Can you work these out from the model? Positions are in its coordinate system, mm. Round coordinates to 2 decimals unless told otherwise and drop trailing zeros. Loops run counter-clockwise (first coordinate to the right, second up) from the corner with the lowest first, then second, coordinate; pieces in that order, holes last.
```python
from build123d import *

# Parameters (mm, degrees)
F1_DEPTH = 14
F2_R     = 8
F2_R_2   = 3.25
F3_DEPTH = 14.001


with BuildPart() as f1:
    # F0 (on Front) → F1 (new body)
    with BuildSketch(Plane.XZ):
        with BuildLine():
            Line((-46.5, -24.5), (46.5, -24.5))
            Line((46.5, -24.5), (46.5, 19.5))
            ThreePointArc((46.5, 19.5), (45.035534, 23.035534), (41.5, 24.5))
            Line((41.5, 24.5), (-41.5, 24.5))
            ThreePointArc((-41.5, 24.5), (-45.035534, 23.035534), (-46.5, 19.5))
            Line((-46.5, 19.5), (-46.5, -24.5))
        make_face()
    extrude(amount=F1_DEPTH)

    # F2 (on face) → F3 (cut, through all)
    with BuildSketch(Plane.XZ.offset(14)):
        Circle(F2_R)
        with Locations((-17, -6)):
            Circle(F2_R_2)
        with Locations((-25, 16)):
            Circle(F2_R_2)
        with Locations((25, 16)):
            Circle(F2_R_2)
        with Locations((17, -6)):
            Circle(F2_R_2)
    extrude(amount=-F3_DEPTH, mode=Mode.SUBTRACT)


solid = f1.part
```
(1) We'd pull the mould along Z, two halves only. Please class faces 1 (the cylindrical face through (24.577, -7.098, 19.222)), 2 (the cylindrical face through (-45, -6.9, 23.07)), 3 (the flat face through (46.5, -7, -3)), 4 (the cylindrical face through (-20.247, -7.098, -5.857)): released by +Z, released by -Z, zero draft, split by the parting line, or undercut.
(2) Suppose I cut it at A-A (x = -25). Write out the boundary of the cut face in (y, z).
(3) Suppose I cut it at C-C (z = -6). Write out the boundary of the cut face in (x, y), then the cut area to 3 significant figures.
(4) Suppose I cut it at D-D (z = 2.5). Write out the boundary of the cut face in (x, y).
(5) If I drill on line 1 (Z direction, x = -25, y = -11); line 2 (Z direction, x = -17, y = -4.75); line 3 (X direction, y = -3, z = 17.5), over which ranges is the centre line in solid material (lowest first)?
(6) Suppose I cut it at B-B (y = -5.5). Write out the boundary of the cut face in (x, z), then the cut area to 3 significant figures.
Check result:
1. face 1: undercut
1. face 2: released by +Z
1. face 3: zero draft
1. face 4: undercut
2. outline: (-14, -24.5) - (0, -24.5) - (0, 12.75) - (-14, 12.75) - close; (-14, 19.25) - (0, 19.25) - (0, 24.5) - (-14, 24.5) - close
3. outline: (-46.5, -14) - (-20.25, -14) - (-20.25, 0) - (-46.5, 0) - close; (-13.75, -14) - (-5.29, -14) - (-5.29, 0) - (-13.75, 0) - close; (5.29, -14) - (13.75, -14) - (13.75, 0) - (5.29, 0) - close; (20.25, -14) - (46.5, -14) - (46.5, 0) - (20.25, 0) - close
3. area: 972 mm2
4. outline: (-46.5, -14) - (-7.6, -14) - (-7.6, 0) - (-46.5, 0) - close; (7.6, -14) - (46.5, -14) - (46.5, 0) - (7.6, 0) - close
5. line 1: z = -24.5 to 12.75, 19.25 to 24.5
5. line 2: z = -24.5 to -9.25, -2.75 to 24.5
5. line 3: x = -46.5 to -27.88, -22.12 to 22.12, 27.88 to 46.5
6. outline: (-46.5, -24.5) - (46.5, -24.5) - (46.5, 19.5) arc R5 ccw to (41.5, 24.5) - (-41.5, 24.5) arc R5 ccw to (-46.5, 19.5) - close; hole circle Ø6.5 at (-25, 16); hole circle Ø6.5 at (-17, -6); hole circle Ø16 at (0, 0); hole circle Ø6.5 at (17, -6); hole circle Ø6.5 at (25, 16)
6. area: 4,210 mm2
